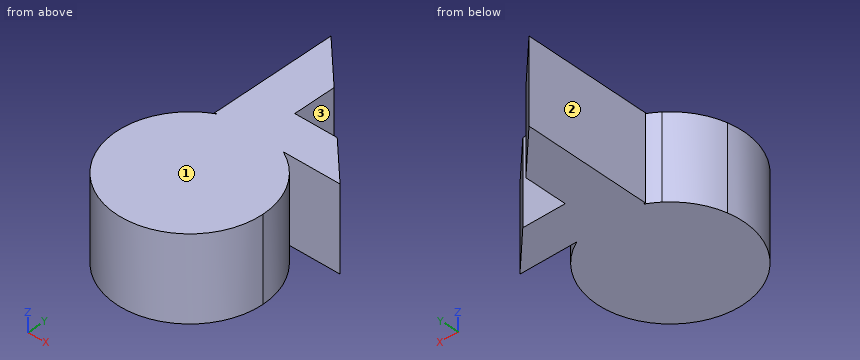
```python
from build123d import *

# Parameters (mm, degrees)
F1_DEPTH = 40


with BuildPart() as f1:
    # F0 (on Top) → F1 (new body)
    with BuildSketch(Plane.XY):
        with BuildLine():
            ThreePointArc((3.942309171, -3.5829284162), (-4.2047941466, -12.6023770601), (-8.7761012616, -23.8642107282))
            Line((-8.7761012616, -23.8642107282), (3.942309171, -23.8642107282))
            Line((3.942309171, -23.8642107282), (3.942309171, -3.5829284162))
        make_face()
        with BuildLine():
            Line((3.942309171, -23.8642107282), (-8.7761012616, -23.8642107282))
            ThreePointArc((-8.7761012616, -23.8642107282), (21.7601480197, -66.0023779885), (60.4471145943, -31.1971157789))
            ThreePointArc((60.4471145943, -31.1971157789), (55.2826725913, -12.8984961859), (41.3134300795, 0))
            Line((41.3134300795, 0), (9.5807991091, 0))
            ThreePointArc((9.5807991091, 0), (6.6758729332, -1.6566268442), (3.942309171, -3.5829284162))
            Line((3.942309171, -3.5829284162), (3.942309171, -23.8642107282))
        make_face()
        with BuildLine():
            ThreePointArc((41.3134300795, 0), (25.4471145943, 3.8028842211), (9.5807991091, 0))
            Line((9.5807991091, 0), (41.3134300795, 0))
        make_face()
        with BuildLine():
            Line((8.4807705134, 0), (9.5807991091, 0))
            ThreePointArc((9.5807991091, 0), (25.4471145943, 3.8028842211), (41.3134300795, 0))
            Line((41.3134300795, 0), (68.4807705134, 0))
            Line((68.4807705134, 0), (49.6739435196, 18.8068269938))
            Line((49.6739435196, 18.8068269938), (29.3806760758, 18.8068269938))
            Line((29.3806760758, 18.8068269938), (29.3806760758, 39.1000944376))
            Line((29.3806760758, 39.1000944376), (8.4807705134, 60))
            Line((8.4807705134, 60), (8.4807705134, 0))
        make_face()
    extrude(amount=F1_DEPTH)


solid = f1.part
```
Work out the finished part from the listing and answer in its coordinate system (mm). Face numbers are marked on the shaded views. A direction names the side the tool comes from. Give positions to 0.01 mm unless a question says otherwise; leave off trailing zeros. Loops run counter-clockwise (first coordinate to the right, second up) from the corner with the lowest first, then second, coordinate; pieces in that order, holes last. Notation, with made-up numbers: (-2, 56) -> (13, 56) arc R28 cw to (13, 87) -> close; hole circle Ø3 at (-2, 16.5). An arc over 180 degrees is marked (long way). Write item = value, one per line. Start each with the question number.
(1) Which of the six approach directions +Z, -Z, +X, -X, +Y, -Y give full straight-line access (tool end or side, diameter ignored) to the marked faces 1, 2 and 3?
(2) Find section A-A on x = 54. Give the vertices of the cut face in (y, z).
(3) Find section B-B on z = 28. Give the vertices of the cut face in (x, y), and give its area (3 significant figures).
(4) Find the intervals of material crossed by probe 1 along Y at (x, z) = (55.5, 20); probe 2 along X at (y, z) = (-40, 15.5); probe 3 along X at (y, z) = (51, 10), in increasing order. Write a range as from..to.
(5) Find section D-D on x = 36.5. Give the vertices of the cut face in (y, z), and give its area (3 significant figures).
(6) Find section C-C on y = 23. Give the vertices of the cut face in (x, z).
(7) Given pin 1 Ø8 at (x, z) = (58.5, 22) entering from -Y; pin 2 Ø4 at (y, z) = (-16.5, 20.5) entering from -X; pin 3 Ø8 at (y, z) = (13, 27.5) entering from -X, each flat-ended and moving along its own axis, determine where each tip first touches the part or whether it passes through.
From the geometry:
q1.face_1 = +Z, +X, -X, +Y, -Y
q1.face_2 = +Z, -Z, -X, +Y
q1.face_3 = +Z, -Z, +X, +Y
q2.outline = (-51.44, 0) -> (-10.96, 0) -> (-10.96, 40) -> (-51.44, 40) -> close; (0, 0) -> (14.48, 0) -> (14.48, 40) -> (0, 40) -> close
q3.outline = (8.48, 0) -> (9.58, 0) arc R35 ccw (long way) to (41.31, 0) -> (68.48, 0) -> (49.67, 18.81) -> (29.38, 18.81) -> (29.38, 39.1) -> (8.48, 60) -> close
q3.area = 5,360 mm^2
q4.probe_1 = -49.14..-13.26, 0..12.98
q4.probe_2 = -8.43..59.32
q4.probe_3 = 8.48..17.48
q5.outline = (-64.41, 0) -> (18.81, 0) -> (18.81, 40) -> (-64.41, 40) -> close
q5.area = 3,330 mm^2
q6.outline = (8.48, 0) -> (29.38, 0) -> (29.38, 40) -> (8.48, 40) -> close
q7.pin_1 = -50.71
q7.pin_2 = -7.17
q7.pin_3 = 8.48
